```python
from build123d import *

# Parameters (mm, degrees)
SKETCH1_W          = 10
SKETCH1_H          = 20
SKETCH2_R          = 5
CUT_EXTRUDE1_DEPTH = 20
CUT_EXTRUDE2_DEPTH = 5
CUT_EXTRUDE3_DEPTH = 5


with BuildPart() as part:
    # Sketch1 → Revolve1 (revolve)
    with BuildSketch(Plane.XY):
        with Locations((5, 10)):
            Rectangle(SKETCH1_W, SKETCH1_H)
    revolve(axis=Axis((0, 0, 0), (0, 1, 0)))

    # Sketch2 → Cut-Extrude1 (cut)
    with BuildSketch(Plane(origin=(0, 20, 0), x_dir=(1, 0, 0), z_dir=(0, 1, 0))):
        Circle(SKETCH2_R)
    extrude(amount=-CUT_EXTRUDE1_DEPTH, mode=Mode.SUBTRACT)

    # Sketch3 → Cut-Extrude2 (cut)
    with BuildSketch(Plane(origin=(0, 20, 0), x_dir=(1, 0, 0), z_dir=(0, 1, 0))):
        with BuildLine():
            Line((-10, 0), (-5, 0))
            ThreePointArc((-5, 0), (0, 5), (5, 0))
            Line((5, 0), (10, 0))
            ThreePointArc((10, 0), (0, 10), (-10, 0))
        make_face()
    extrude(amount=-CUT_EXTRUDE2_DEPTH, mode=Mode.SUBTRACT)

    # Sketch4 → Cut-Extrude3 (cut)
    with BuildSketch(Plane.XZ):
        with BuildLine():
            Line((-10, 0), (-5, 0))
            ThreePointArc((-5, 0), (0, -5), (5, 0))
            Line((5, 0), (10, 0))
            ThreePointArc((10, 0), (0, -10), (-10, 0))
        make_face()
    extrude(amount=-CUT_EXTRUDE3_DEPTH, mode=Mode.SUBTRACT)


solid = part.part
```
For this review, take the finished solid that the model builds, in its own axes (mm). A direction names the side the tool comes from. Round coordinates to 2 decimals unless told otherwise and drop trailing zeros. Write each loop counter-clockwise with the first axis right and the second up, starting at its lowest first coordinate (ties: lowest second). Pieces come first, ordered by that corner, then holes. Notation, with made-up numbers: (-15.75, 36) -> (38.25, 36) arc R15 cw to (38.25, 63) -> close; hole circle Ø9 at (-8, -15.5). An arc over 180 degrees is marked (long way). Use one line per item in the form item = value.
1) Take a section at A-A, the plane x = 0. Write out the cut boundary in (y, z), and give its area (3 significant figures).
Found:
outline = (0, 5) -> (20, 5) -> (20, 10) -> (0, 10) -> close; (5, -10) -> (15, -10) -> (15, -5) -> (5, -5) -> close
area = 150 mm2
2) Tool access review of faces 5 (the flat face through (0, 20, 6)), 6 (the flat face through (-8, 2, 0)), 7 (the flat face through (-8, 18, 0)): name each direction out of +Z, -Z, +X, -X, +Y, -Y from which nothing blocks a thin tool from reaching the whole face with its end or side.
Found:
face_5 = +Z, -Z, +X, -X, +Y
face_6 = -Z, +X, -X, -Y
face_7 = -Z, +X, -X, +Y
3) To check wall thickness, follow L1, parallel to Z at x = 0, y = 7.25; L2, parallel to Y at x = 5.25, z = -0.5. State the ranges of each line that lie inside material, in increasing order. Write a range as from..to.
Found:
L1 = -10..-5, 5..10
L2 = 5..15
4) Take a section at D-D, the plane y = 2.75. Write out the cut boundary in (x, z), and give its area (3 significant figures).
Found:
outline = (-10, 0) -> (-5, 0) arc R5 cw to (5, 0) -> (10, 0) arc R10 ccw to start
area = 118 mm2
5) Take a section at C-C, the plane y = 8.5. Write out the cut boundary in (x, z).
Found:
outline = circle Ø20 at (0, 0); hole circle Ø10 at (0, 0)
6) Take a section at B-B, the plane z = 2.5. Write out the cut boundary in (x, y).
Found:
outline = (-9.68, 0) -> (-4.33, 0) -> (-4.33, 20) -> (-9.68, 20) -> close; (4.33, 0) -> (9.68, 0) -> (9.68, 20) -> (4.33, 20) -> close
7) Clearance check with flat-ended pins moving along their axes: pin 1 (2 mm diameter, centred on y = 15, z = -6.5, fed in from +X); pin 2 (1.5 mm diameter, centred on x = -8, y = 17, fed in from -Z); pin 3 (4 mm diameter, centred on x = 6.5, y = 3.5, fed in from -Z). State where each tip first meets the part, or that it passes through.
Found:
pin_1 = 8.35
pin_2 = 0
pin_3 = -8.56
8) Mouldability with a two-part tool opening along Z and no side actions: class faces 1 (the cylindrical face through (-1.08, 10.14, 4.88)), 2 (the flat face through (0, 5, -6)), 3 (the cylindrical face through (-2.17, 10.14, 9.76)), 4 (the flat face through (7, 2, 0)) as +Z half, -Z half, draft (parallel to the pull), parting line (faces both ways), or undercut.
Found:
face_1 = undercut
face_2 = draft
face_3 = parting line
face_4 = -Z half
